Check sheet for the drawn part. Datum: minimum x, y, z corner. Units: mm. A direction names the side the tool comes from. Round coordinates to 2 decimals unless told otherwise and drop trailing zeros. Order: outer loops, then holes, each group sorted by start corner. A loop starts at its lowest first (then second) coordinate and runs counter-clockwise, first axis right, second up. Notation, with made-up numbers: (-38, -1) - (9, -1) arc R28 ccw to (9, 26) - close; hole circle Ø9 at (25, 63.5). An arc over 180 degrees is marked (long way). Write each question's results on one line, items separated by ' | '.
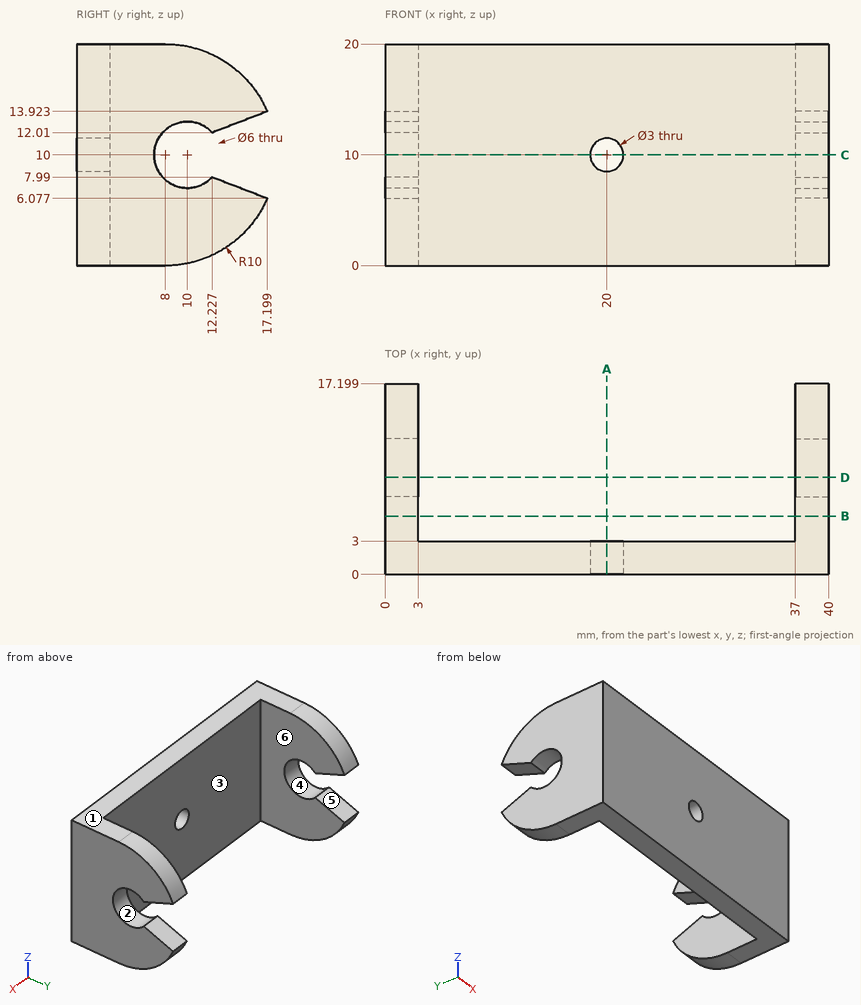
(1) Access from +Z, -Z, +X, -X, +Y, -Y to the whole of each face (thin tool, end or side, straight path). Record for the marked faces 4, 5 and 6.
Answers follow:
face 4: +X, -X | face 5: +X, -X, +Y | face 6: +Z, -Z, +Y
(2) Section check D-D (y = 8.75). Record the cut outline in (x, z).
Answers follow:
outline: (0, 0.03) - (3, 0.03) - (3, 7.27) - (0, 7.27) - close; (0, 12.73) - (3, 12.73) - (3, 19.97) - (0, 19.97) - close; (37, 0.03) - (40, 0.03) - (40, 7.27) - (37, 7.27) - close; (37, 12.73) - (40, 12.73) - (40, 19.97) - (37, 19.97) - close
(3) Section check A-A (x = 20). Record the cut outline in (y, z), then the cut area to 3 significant figures.
Answers follow:
outline: (0, 0) - (3, 0) - (3, 8.5) - (0, 8.5) - close; (0, 11.5) - (3, 11.5) - (3, 20) - (0, 20) - close | area: 51.0 mm²
(4) Material ranges on line 1 (X direction, y = 6.75, z = 10.5); line 2 (X direction, y = 0.8, z = 10); line 3 (Y direction, x = 39.35, z = 10), recorded low to high.
Answers follow:
line 1: 0 to 3, 37 to 40 | line 2: 0 to 18.5, 21.5 to 40 | line 3: 0 to 7
(5) Section check B-B (y = 5.25). Record the cut outline in (x, z), then the cut area to 3 significant figures.
Answers follow:
outline: (0, 0) - (3, 0) - (3, 20) - (0, 20) - close; (37, 0) - (40, 0) - (40, 20) - (37, 20) - close | area: 120 mm²
(6) Section check C-C (z = 10). Record the cut outline in (x, y).
Answers follow:
outline: (0, 0) - (18.5, 0) - (18.5, 3) - (3, 3) - (3, 7) - (0, 7) - close; (21.5, 0) - (40, 0) - (40, 7) - (37, 7) - (37, 3) - (21.5, 3) - close
(7) Draft check along Z on the marked faces 1, 2 and 3. Enter one of: released by +Z, released by -Z, zero draft, split by the parting line, or undercut.
Answers follow:
face 1: released by +Z | face 2: undercut | face 3: zero draft
(8) Depth check by flat-ended pin: pin 1 Ø3.5 at (y, z) = (10, 10) entering from -X; pin 2 Ø5 at (x, z) = (9.5, 16) entering from -Y; pin 3 Ø5 at (x, z) = (16.5, 7.5) entering from +Y. Enter the tip coordinate at first touch or a pass-through.
Answers follow:
pin 1: through | pin 2: y = 0 | pin 3: y = 3
